For this review, take the finished solid that the model builds, in its own axes (mm). Face numbers are marked on the shaded views. Round coordinates to 2 decimals unless told otherwise and drop trailing zeros. Order: outer loops, then holes, each group sorted by start corner. A loop starts at its lowest first (then second) coordinate and runs counter-clockwise, first axis right, second up. Notation, with made-up numbers: M 52.5,25 L 56.5,25 A27 ccw 56.5,48 Z; hole C -1,82.25 d11. An arc over 180 degrees is marked long. Put each result on its own line as item: value.
from build123d import *

# Parameters (mm, degrees)
F2_SIZE  = 1
F4_R     = 5
F5_R     = 8.75
F6_DEPTH = 52.501


# Not quite as in the source:
# - two fillets or chamfers of one size are made in one step


with BuildPart() as f1:
    # F0 (on Front) → F1 (revolve)
    with BuildSketch(Plane.XZ):
        Polygon((-3.5, 21.75), (35.7057713659, 21.75), (52.5, 26.25), (52.5, 27.84), (50.7274746578, 30.15), (31.5788313746, 30.15), (17, 37.7090089023), (17, 70), (0, 70), (0, 38.7), (6, 38.7), (6, 31.5), (0, 31.5), (0, 28), (-3.5, 28), align=None)
    revolve(axis=Axis((44.485598996, 0, 0), (1, 0, 0)))

    # F2
    f2_edges = [f1.edges().sort_by_distance(p)[0] for p in [
        (17, 0, -70),
        (0, 0, -70),
        (0, 0, -31.5),
        (0, 0, -28),
    ]]
    chamfer(f2_edges, length=F2_SIZE)

    # F4
    f4_edges = [f1.edges().sort_by_distance(p)[0] for p in [
        (17, 0, -37.709009),
        (31.578831, 0, -30.15),
    ]]
    fillet(f4_edges, radius=F4_R)

    # F5 (on face) → F6 (cut, through all)
    with BuildSketch(Plane(origin=(0, 0, 0), x_dir=(0, -1, 0), z_dir=(-1, 0, 0))):
        with Locations((0, 52.5)):
            Circle(F5_R)
        with Locations((-52.5, 0)):
            Circle(F5_R)
        with Locations((52.5, 0)):
            Circle(F5_R)
        with Locations((0, -52.5)):
            Circle(F5_R)
    extrude(amount=-F6_DEPTH, mode=Mode.SUBTRACT)


solid = f1.part
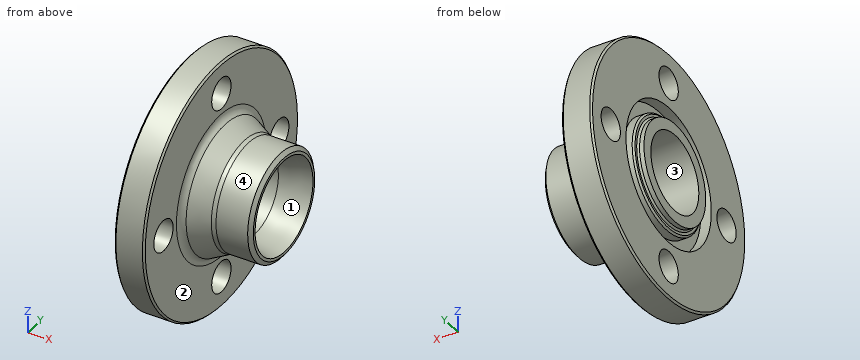
(1) Add section A-A on z = 0. State how many separate pieces and enclosed holes the cut face has, then the cut area to 3 significant figures.
A:
separate pieces: 4
enclosed holes: 0
area: 1,630 mm2
(2) Draft analysis for pull direction Y (two halves, no side actions). For the marked faces 1, 2, 3 and 4, state which applies: released by +Y, released by -Y, zero draft, split by the parting line, or undercut.
A:
face 1: undercut
face 2: zero draft
face 3: undercut
face 4: split by the parting line
(3) Add section C-C on x = 42.5. Give the boundary of the cut face in (y, z), then the cut area to 3 significant figures.
A:
outline: C 0,0 d60.3; hole C 0,0 d47.14
area: 1,110 mm2
(4) Insertion check: pin 1 Ø6 at (y, z) = (-22, 48) entering from +X; pin 2 Ø4 at (x, z) = (18, -11.5) entering from +Y; pin 3 Ø10 at (x, y) = (24, -3) entering from -Z. Each pin has a flat end and moves straight along its axis. Give the tip position at first contact, or say it passes through.
A:
pin 1: stops at x = 17
pin 2: stops at y = 69.08
pin 3: stops at z = -36.64
(5) To check wall thickness, follow L1, parallel to Z at x = 5, y = 0; L2, parallel to Z at x = 8.25, y = 0; L3, parallel to X at y = 19.5, z = -49. State the ranges of each line that lie inside material, in increasing order.
A:
L1: z = -70 to -61.25, -43.75 to -38.7, -31.5 to -21.75, 21.75 to 31.5, 38.7 to 43.75, 61.25 to 70
L2: z = -70 to -61.25, -43.75 to -21.75, 21.75 to 43.75, 61.25 to 70
L3: x = 0 to 17
